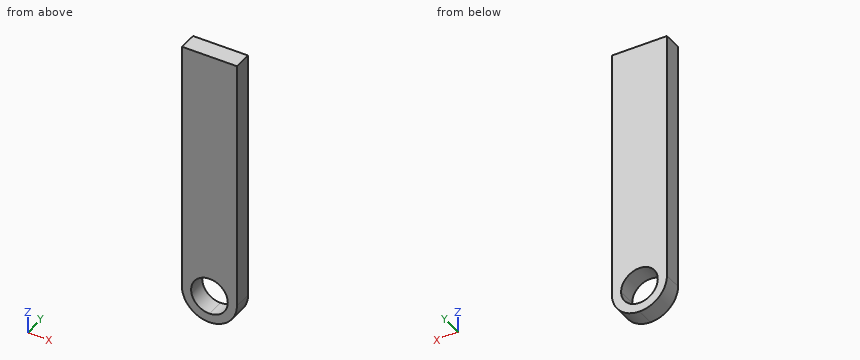
```python
from build123d import *

# Parameters (mm, degrees)
F1_DEPTH = 3.175
F2_R     = 4.76249


# Not quite as in the source:
# - a fillet or chamfer is up to 0.001 mm smaller than in the source, because OpenCascade refuses the exact size


with BuildPart() as f1:
    # F0 (on Front) → F1 (new body)
    with BuildSketch(Plane.XZ):
        Polygon((0, 3.175), (0, 0), (0, -45.3541763127), (4.7625, -45.3541763127), (9.525, -45.3541763127), (9.525, 3.175), align=None)
        with BuildLine():
            ThreePointArc((7.9375, -40.5916763127), (7.0075640303, -42.836740343), (4.7625, -43.7666763127))
            ThreePointArc((4.7625, -43.7666763127), (2.5174359697, -38.3466122824), (7.9375, -40.5916763127))
        make_face(mode=Mode.SUBTRACT)
    extrude(amount=F1_DEPTH)

    # F2 (radius 4.7625 in the source; OpenCascade refuses exactly that, so slightly less here)
    f2_edges = [f1.edges().sort_by_distance(p)[0] for p in [
        (0, -1.5875, -45.354176),
        (9.525, -1.5875, -45.354176),
    ]]
    fillet(f2_edges, radius=F2_R)


solid = f1.part
```
Verification items for the finished model (mm, model axes). Round coordinates to 2 decimals unless told otherwise and drop trailing zeros. Write each loop counter-clockwise with the first axis right and the second up, starting at its lowest first coordinate (ties: lowest second). Pieces come first, ordered by that corner, then holes.
1. Section check C-C on z = -39. Enter the section's corners in (x, y) (3 decimals).
2. Scan lines: L1, parallel to Z at x = 4.75, y = -2.25 (3 decimals); L2, parallel to X at y = -0.4, z = -39 (3 decimals); L3, parallel to Z at x = 2.75, y = -0.7 (3 decimals). Record each from-to range of solid material in increasing order.
3. Section check B-B on x = 6.5. Enter the section's corners in (y, z) (3 decimals), plus the area to 3 significant figures.
4. Gauge pin test, flat ends, axial feed: P1, Ø1.5, axis at x = 2.5, y = -1, coming from the -Z side; P2, Ø5.5, axis at x = 4.76, z = -40.59, coming from the -Y side. Record the tip position at first contact, or that the pin passes through.
Answer:
1. outline: (0, -3.175) - (2.015, -3.175) - (2.015, 0) - (0, 0) - close; (7.51, -3.175) - (9.525, -3.175) - (9.525, 0) - (7.51, 0) - close
2. L1: z = -45.354 to -43.767, -37.417 to 3.175
2. L2: x = 0 to 2.015, 7.51 to 9.525
2. L3: z = -44.908 to -43.047, -38.136 to 3.175
3. outline: (-3.175, -45.026) - (0, -45.026) - (0, -43.249) - (-3.175, -43.249) - close; (-3.175, -37.934) - (0, -37.934) - (0, 3.175) - (-3.175, 3.175) - close
3. area: 136 mm2
4. P1: stops at z = -45.11
4. P2: passes through
